Check sheet for the modelled part. Datum: model origin and axes. Units: mm. Round coordinates to 2 decimals unless told otherwise and drop trailing zeros. Order: outer loops, then holes, each group sorted by start corner. A loop starts at its lowest first (then second) coordinate and runs counter-clockwise, first axis right, second up. Notation, with made-up numbers: M 54.25,29.25 L 64.25,29.25 A31 cw 64.25,59.25 Z; hole C 89.5,23 d9. An arc over 180 degrees is marked long. One line per item, written item: value. Start each with the question number.
(1) Cross-section at B-B, the plane z = 5.5. Enter the section's corners in (x, y).
(2) Depth check by flat-ended pin: pin 1 Ø12.5 at (x, z) = (-91, 8) entering from -Y; pin 2 Ø12.5 at (y, z) = (143.5, 16.5) entering from -X; pin 3 Ø12.5 at (y, z) = (192.5, 15) entering from +X. Enter the tip coordinate at first touch or a pass-through.
(3) Cross-section at C-C, the plane y = 1141.5. Enter the section's corners in (x, z).
(4) Cross-section at A-A, the plane x = -140. Enter the section's corners in (y, z), and give its area (3 significant figures).
(5) Thickness scan on L1, parallel to Y at x = -112, z = 21.75; L2, parallel to X at y = 494.5, z = 12; L3, parallel to X at y = 1225.5, z = 4. Record the ranges inside material, lowest first.
(6) Cross-section at D-D, the plane x = 248. Enter the section's corners in (y, z), and give its area (3 significant figures).
from build123d import *

# Parameters (mm, degrees)
F0_W     = 50.8
F0_H     = 482.6
F0_W_2   = 23.167712307
F0_H_2   = 76.2
F0_H_3   = 145.5220067978
F0_H_4   = 311.2254058838
F0_H_5   = 165.2207044601
F0_W_3   = 285.75
F0_H_6   = 38.4318828583
F1_DEPTH = 25.4


with BuildPart() as f1:
    # F0 (on Top) → F1 (new body)
    with BuildSketch(Plane.XY):
        with Locations((0, 241.3)):
            Rectangle(F0_W, F0_H)
        with Locations((-36.9838561535, 520.7)):
            Rectangle(F0_W_2, F0_H_2)
        with Locations((0, 520.7)):
            Rectangle(F0_W, F0_H_2)
        with Locations((36.9838561535, 520.7)):
            Rectangle(F0_W_2, F0_H_2)
        with Locations((-36.9838561535, 631.5610033989)):
            Rectangle(F0_W_2, F0_H_3)
        with Locations((36.9838561535, 631.5610033989)):
            Rectangle(F0_W_2, F0_H_3)
        Polygon((-48.567712307, 704.3220067978), (-25.4, 704.3220067978), (-25.4, 1015.5474126816), (-177.8, 1015.5474126816), (-177.8, 558.8), (-48.567712307, 558.8), align=None)
        with Locations((0, 859.9347097397)):
            Rectangle(F0_W, F0_H_4)
        Polygon((25.4, 1015.5474126816), (25.4, 704.3220067978), (48.567712307, 704.3220067978), (48.567712307, 558.8), (177.8, 558.8), (177.8, 1015.5474126816), align=None)
        with Locations((0, 1098.1577649117)):
            Rectangle(F0_W, F0_H_5)
        with Locations((-168.275, 1199.9840585709)):
            Rectangle(F0_W_3, F0_H_6)
        with Locations((0, 1199.9840585709)):
            Rectangle(F0_W, F0_H_6)
        with Locations((168.275, 1199.9840585709)):
            Rectangle(F0_W_3, F0_H_6)
        with Locations((0, 1460.5)):
            Rectangle(F0_W, F0_H)
        with Locations((0, 631.5610033989)):
            Rectangle(F0_W, F0_H_3)
    extrude(amount=F1_DEPTH)


solid = f1.part
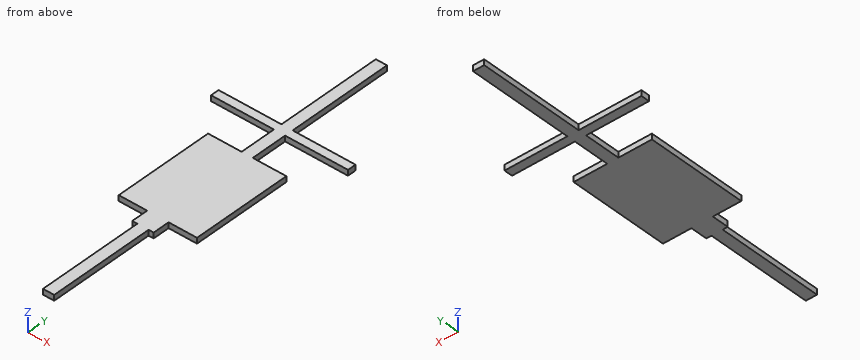
Values found:
1. outline: M -311.15,1180.77 L -25.4,1180.77 L -25.4,1015.55 L -177.8,1015.55 L -177.8,558.8 L -48.57,558.8 L -48.57,482.6 L -25.4,482.6 L -25.4,0 L 25.4,0 L 25.4,482.6 L 48.57,482.6 L 48.57,558.8 L 177.8,558.8 L 177.8,1015.55 L 25.4,1015.55 L 25.4,1180.77 L 311.15,1180.77 L 311.15,1219.2 L 25.4,1219.2 L 25.4,1701.8 L -25.4,1701.8 L -25.4,1219.2 L -311.15,1219.2 Z
2. pin 1: y = 558.8
2. pin 2: x = -25.4
2. pin 3: x = 25.4
3. outline: M -25.4,0 L 25.4,0 L 25.4,25.4 L -25.4,25.4 Z
4. outline: M 558.8,0 L 1015.55,0 L 1015.55,25.4 L 558.8,25.4 Z; M 1180.77,0 L 1219.2,0 L 1219.2,25.4 L 1180.77,25.4 Z
4. area: 12,600 mm^2
5. L1: 558.8 to 1015.55, 1180.77 to 1219.2
5. L2: -48.57 to 48.57
5. L3: -25.4 to 25.4
6. outline: M 1180.77,0 L 1219.2,0 L 1219.2,25.4 L 1180.77,25.4 Z
6. area: 976 mm^2
